Geometry: final body of the model. Coordinates: model frame, mm. Face numbers are marked on the shaded views. A direction names the side the tool comes from. Give positions to 0.01 mm unless a question says otherwise; leave off trailing zeros. Write each loop counter-clockwise with the first axis right and the second up, starting at its lowest first coordinate (ties: lowest second). Pieces come first, ordered by that corner, then holes. Notation, with made-up numbers: M 2.5,-12.5 L 36.5,-12.5 A18 cw 36.5,-2.5 Z; hole C -37.5,72.25 d8. An arc over 180 degrees is marked long. Use a Markdown table: item, result. Add a question column.
(1) Cut plane A-A (y = 0). Output: boundary loops of the cut face in (x, z), plus the area to 3 significant figures.
(2) Cut plane D-D (y = -6). Output: boundary loops of the cut face in (x, z).
(3) Pin query (flat end, axial travel): pin 1 Ø2 at (x, y) = (9, -13.5) entering from +Z; pin 2 Ø2 at (x, z) = (10.5, 2) entering from +Y. Return the tip coordinate at first contact, or that it passes through.
(4) Material intervals for L1, parallel to Y at x = 8.5, z = 1.1; L2, parallel to X at y = -1, z = 1.65; L3, parallel to Y at x = 8.5, z = 3.7, sorted ascending.
(5) Draft query along X for the marked faces 4, 5, 6 and 7. Return one class per face: released by +X, released by -X, zero draft, split by the parting line, or undercut.
(6) Cut plane B-B (x = 8.5). Output: boundary loops of the cut face in (y, z), plus the area to 3 significant figures.
(7) Cut plane C-C (x = 0). Output: boundary loops of the cut face in (y, z).
(8) Reachability of the marked faces 1, 2 and 3 from +Z, -Z, +X, -X, +Y, -Y: full face, straight path, thin tool, end or side. Return the list, or none.
```python
from build123d import *

# Parameters (mm, degrees)
ESQUISSE1_R                                        = 21.4
BOSS_EXTRU_1_DEPTH                                 = 6
ESQUISSE2_R                                        = 12.5
ENL_V_MAT_EXTRU_1_DEPTH                            = 3
CHAMBRAGE_POUR_VIS_T_TE_HEXAGONALE_M31_D           = 3.4
CHAMBRAGE_POUR_VIS_T_TE_HEXAGONALE_M31_DEPTH       = 8
CHAMBRAGE_POUR_VIS_T_TE_HEXAGONALE_M31_CBORE_D     = 6.5
CHAMBRAGE_POUR_VIS_T_TE_HEXAGONALE_M31_CBORE_DEPTH = 3.4
CHAMBRAGE_POUR_VIS_T_TE_HEXAGONALE_M31_TIP         = 1.021463052


with BuildPart() as part:
    # Esquisse1 → Boss.-Extru.1 (new body)
    with BuildSketch(Plane.XY):
        Circle(ESQUISSE1_R)
    extrude(amount=BOSS_EXTRU_1_DEPTH)

    # Esquisse2 → Enlèv. mat.-Extru.1 (cut)
    with BuildSketch(Plane(origin=(0, 0, 0), x_dir=(-1, 0, 0), z_dir=(0, 0, -1))):
        Circle(ESQUISSE2_R)
    extrude(amount=-ENL_V_MAT_EXTRU_1_DEPTH, mode=Mode.SUBTRACT)

    # Chambrage pour vis à tête hexagonale M31
    with Locations(Plane.XY.offset(6)):
        with Locations((-17, 0), (8.5, 14.722431864), (8.5, -14.722431864)):
            CounterBoreHole(CHAMBRAGE_POUR_VIS_T_TE_HEXAGONALE_M31_D / 2, CHAMBRAGE_POUR_VIS_T_TE_HEXAGONALE_M31_CBORE_D / 2, CHAMBRAGE_POUR_VIS_T_TE_HEXAGONALE_M31_CBORE_DEPTH, depth=CHAMBRAGE_POUR_VIS_T_TE_HEXAGONALE_M31_DEPTH)
            with Locations((0, 0, -(CHAMBRAGE_POUR_VIS_T_TE_HEXAGONALE_M31_DEPTH + CHAMBRAGE_POUR_VIS_T_TE_HEXAGONALE_M31_TIP / 2))):  # 118° drill point
                Cone(0, CHAMBRAGE_POUR_VIS_T_TE_HEXAGONALE_M31_D / 2, CHAMBRAGE_POUR_VIS_T_TE_HEXAGONALE_M31_TIP, mode=Mode.SUBTRACT)


solid = part.part
```
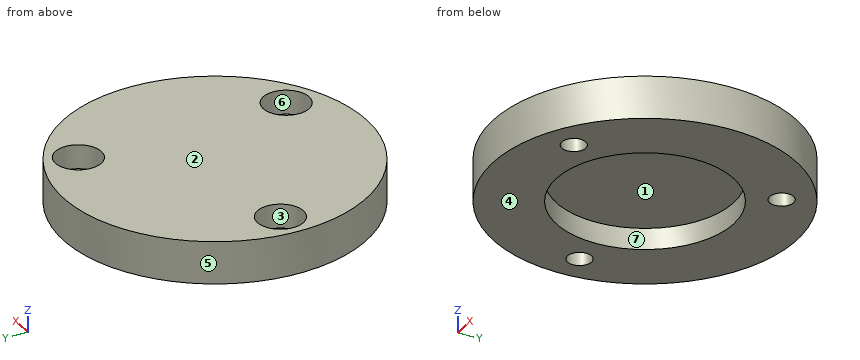
Answer list:
| question | item | result |
|---|---|---|
| 1 | outline | M -21.4,0 L -18.7,0 L -18.7,2.6 L -20.25,2.6 L -20.25,6 L -21.4,6 Z; M -15.3,0 L -12.5,0 L -12.5,3 L 12.5,3 L 12.5,0 L 21.4,0 L 21.4,6 L -13.75,6 L -13.75,2.6 L -15.3,2.6 Z |
| 1 | area | 151 mm² |
| 2 | outline | M -20.54,0 L -10.97,0 L -10.97,3 L 10.97,3 L 10.97,0 L 20.54,0 L 20.54,6 L -20.54,6 Z |
| 3 | pin 1 | z = 2.6 |
| 3 | pin 2 | y = 19.18 |
| 4 | L1 | -19.64 to -16.42, -13.02 to -9.17, 9.17 to 13.02, 16.42 to 19.64 |
| 4 | L2 | -21.38 to -18.37, -15.63 to -12.46, 12.46 to 21.38 |
| 4 | L3 | -19.64 to -17.97, -11.47 to 11.47, 17.97 to 19.64 |
| 5 | face 4 | zero draft |
| 5 | face 5 | split by the parting line |
| 5 | face 6 | undercut |
| 5 | face 7 | undercut |
| 6 | outline | M -19.64,0 L -16.42,0 L -16.42,2.6 L -17.97,2.6 L -17.97,6 L -19.64,6 Z; M -13.02,0 L -9.17,0 L -9.17,3 L 9.17,3 L 9.17,0 L 13.02,0 L 13.02,2.6 L 11.47,2.6 L 11.47,6 L -11.47,6 L -11.47,2.6 L -13.02,2.6 Z; M 16.42,0 L 19.64,0 L 19.64,6 L 17.97,6 L 17.97,2.6 L 16.42,2.6 Z |
| 6 | area | 119 mm² |
| 7 | outline | M -21.4,0 L -12.5,0 L -12.5,3 L 12.5,3 L 12.5,0 L 21.4,0 L 21.4,6 L -21.4,6 Z |
| 8 | face 1 | -Z |
| 8 | face 2 | +Z, +X, -X, +Y, -Y |
| 8 | face 3 | +Z |
